Can you work these out from the model? Positions are in its coordinate system, mm. Give positions to 0.01 mm unless a question says otherwise; leave off trailing zeros. Order: outer loops, then holes, each group sorted by start corner. A loop starts at its lowest first (then second) coordinate and runs counter-clockwise, first axis right, second up. Notation, with made-up numbers: (-32, 34.25) -> (-10, 34.25) arc R25 ccw to (-10, 50.25) -> close; hole circle Ø4 at (-40, 33). An arc over 180 degrees is marked (long way). Answer as a JSON object with one key per item and string values.
```python
from build123d import *

# Parameters (mm, degrees)
PLATE_W                                        = 50
PLATE_H                                        = 50
BOSS_EXTRUDE1_DEPTH                            = 3
CSK_FOR_M3_OVAL_HEAD_MACHINE_SCREW1_AT_2_COUNT = 2
CSK_FOR_M3_OVAL_HEAD_MACHINE_SCREW1_AT_2_PITCH = 42
CSK_FOR_M3_OVAL_HEAD_MACHINE_SCREW1_AT_3_COUNT = 2
CSK_FOR_M3_OVAL_HEAD_MACHINE_SCREW1_AT_3_PITCH = 59.39696962
CSK_FOR_M3_OVAL_HEAD_MACHINE_SCREW1_AT_4_COUNT = 2
CSK_FOR_M3_OVAL_HEAD_MACHINE_SCREW1_AT_4_PITCH = 42
F_24_0_24_DIAMETER_HOLE1_D                     = 24
F_24_0_24_DIAMETER_HOLE1_ON_FACE_2_D           = 24
F_24_0_24_DIAMETER_HOLE1_ON_FACE_3_D           = 24
CSK_FOR_M3_OVAL_HEAD_MACHINE_SCREW2_AT_2_COUNT = 2
CSK_FOR_M3_OVAL_HEAD_MACHINE_SCREW2_AT_2_PITCH = 31
CSK_FOR_M3_OVAL_HEAD_MACHINE_SCREW2_AT_3_COUNT = 2
CSK_FOR_M3_OVAL_HEAD_MACHINE_SCREW2_AT_3_PITCH = 43.840620434
CSK_FOR_M3_OVAL_HEAD_MACHINE_SCREW2_AT_4_COUNT = 2
CSK_FOR_M3_OVAL_HEAD_MACHINE_SCREW2_AT_4_PITCH = 31


with BuildPart() as part:
    # Plate → Boss-Extrude1 (new body)
    with BuildSketch(Plane(origin=(0, 0, 0), x_dir=(1, 0, 0), z_dir=(0, 1, 0))):
        Rectangle(PLATE_W, PLATE_H)
    extrude(amount=BOSS_EXTRUDE1_DEPTH)

    # Sketch3 → CSK for M3 Oval Head Machine Screw1 (revolve, cut)
    with BuildSketch(Plane(origin=(-21, 3, 21), x_dir=(0, 0, 1), z_dir=(1, 0, 0))):
        Polygon((0, 0), (0, 3), (1.8, 3), (1.8, 1.35), (3.15, 0), align=None)
    csk_for_m3_oval_head_machine_screw1 = revolve(axis=Axis((-21, 9.35, 21), (0, -1, 0)), mode=Mode.SUBTRACT)

    # CSK for M3 Oval Head Machine Screw1 at 2: CSK for M3 Oval Head Machine Screw1 ×2
    with Locations(*[(0, 0, -i * CSK_FOR_M3_OVAL_HEAD_MACHINE_SCREW1_AT_2_PITCH) for i in range(1, CSK_FOR_M3_OVAL_HEAD_MACHINE_SCREW1_AT_2_COUNT)]):
        add(csk_for_m3_oval_head_machine_screw1, mode=Mode.SUBTRACT)

    # CSK for M3 Oval Head Machine Screw1 at 3: CSK for M3 Oval Head Machine Screw1 ×2
    with Locations(*[Vector(0.707106781, 0, -0.707106781) * (i * CSK_FOR_M3_OVAL_HEAD_MACHINE_SCREW1_AT_3_PITCH) for i in range(1, CSK_FOR_M3_OVAL_HEAD_MACHINE_SCREW1_AT_3_COUNT)]):
        add(csk_for_m3_oval_head_machine_screw1, mode=Mode.SUBTRACT)

    # CSK for M3 Oval Head Machine Screw1 at 4: CSK for M3 Oval Head Machine Screw1 ×2
    with Locations(*[(i * CSK_FOR_M3_OVAL_HEAD_MACHINE_SCREW1_AT_4_PITCH, 0, 0) for i in range(1, CSK_FOR_M3_OVAL_HEAD_MACHINE_SCREW1_AT_4_COUNT)]):
        add(csk_for_m3_oval_head_machine_screw1, mode=Mode.SUBTRACT)

    # Ø24.0 (24) Diameter Hole1 (through all)
    with Locations(Plane.ZX.offset(3)):
        with Locations((0, 0)):
            Hole(F_24_0_24_DIAMETER_HOLE1_D / 2)

    # Ø24.0 (24) Diameter Hole1 on face 2 (through all)
    with Locations(Plane(origin=(0, 0, 0), x_dir=(0, 0, -1), z_dir=(0, -1, 0))):
        with Locations((0, 0)):
            Hole(F_24_0_24_DIAMETER_HOLE1_ON_FACE_2_D / 2)

    # Ø24.0 (24) Diameter Hole1 on face 3 (through all)
    with Locations(Plane(origin=(-62.061079299, -166.048748064, 0), x_dir=(0, 0, 1), z_dir=(0, 1, 0))):
        with Locations((0, 0)):
            Hole(F_24_0_24_DIAMETER_HOLE1_ON_FACE_3_D / 2)

    # Sketch6 → CSK for M3 Oval Head Machine Screw2 (revolve, cut)
    with BuildSketch(Plane(origin=(-15.5, 3, -15.5), x_dir=(0, 0, 1), z_dir=(1, 0, 0))):
        Polygon((0, 0), (0, 3), (1.8, 3), (1.8, 1.35), (3.15, 0), align=None)
    csk_for_m3_oval_head_machine_screw2 = revolve(axis=Axis((-15.5, 9.35, -15.5), (0, -1, 0)), mode=Mode.SUBTRACT)

    # CSK for M3 Oval Head Machine Screw2 at 2: CSK for M3 Oval Head Machine Screw2 ×2
    with Locations(*[(i * CSK_FOR_M3_OVAL_HEAD_MACHINE_SCREW2_AT_2_PITCH, 0, 0) for i in range(1, CSK_FOR_M3_OVAL_HEAD_MACHINE_SCREW2_AT_2_COUNT)]):
        add(csk_for_m3_oval_head_machine_screw2, mode=Mode.SUBTRACT)

    # CSK for M3 Oval Head Machine Screw2 at 3: CSK for M3 Oval Head Machine Screw2 ×2
    with Locations(*[Vector(0.707106781, 0, 0.707106781) * (i * CSK_FOR_M3_OVAL_HEAD_MACHINE_SCREW2_AT_3_PITCH) for i in range(1, CSK_FOR_M3_OVAL_HEAD_MACHINE_SCREW2_AT_3_COUNT)]):
        add(csk_for_m3_oval_head_machine_screw2, mode=Mode.SUBTRACT)

    # CSK for M3 Oval Head Machine Screw2 at 4: CSK for M3 Oval Head Machine Screw2 ×2
    with Locations(*[(0, 0, i * CSK_FOR_M3_OVAL_HEAD_MACHINE_SCREW2_AT_4_PITCH) for i in range(1, CSK_FOR_M3_OVAL_HEAD_MACHINE_SCREW2_AT_4_COUNT)]):
        add(csk_for_m3_oval_head_machine_screw2, mode=Mode.SUBTRACT)


solid = part.part
```
1. If we section it at A-A on z = 21: Please give me the cut outline in (x, y).
Worked answers:
{"outline": "(-25, 0) -> (-22.8, 0) -> (-22.8, 1.65) -> (-24.15, 3) -> (-25, 3) -> close; (-19.2, 0) -> (19.2, 0) -> (19.2, 1.65) -> (17.85, 3) -> (-17.85, 3) -> (-19.2, 1.65) -> close; (22.8, 0) -> (25, 0) -> (25, 3) -> (24.15, 3) -> (22.8, 1.65) -> close"}
2. If we mould it in two halves opening along X, with no side actions, what happens to faces 1 (the face through (-17.285, 0.837, 15.266)), 2 (the face through (-6, 0, -11)), 3 (the face through (-25, 1, 0)), 4 (the face through (19.215, 0.837, 20.766))? For each: +X half, -X half, draft (parallel to the pull), parting line (faces both ways), or undercut.
Worked answers:
{"face 1": "undercut", "face 2": "draft", "face 3": "-X half", "face 4": "undercut"}
3. If we section it at C-C on y = 0.9: Count the separate pieces of the cut face and the enclosed holes in it, then the cut area to 3 significant figures.
Worked answers:
{"separate pieces": "1", "enclosed holes": "9", "area": "1,970 mm²"}
4. If we section it at D-D on z = 0: Please give me the cut outline in (x, y), then the cut area to 3 significant figures.
Worked answers:
{"outline": "(-25, 0) -> (-12, 0) -> (-12, 3) -> (-25, 3) -> close; (12, 0) -> (25, 0) -> (25, 3) -> (12, 3) -> close", "area": "78.0 mm²"}
5. Will these pins go through, and if not, where does the flat tip stop? pin 1 Ø4 at (x, z) = (15.5, -15.5) entering from +Y; pin 2 Ø6 at (x, z) = (21, 21) entering from +Y.
Worked answers:
{"pin 1": "y = 1.85", "pin 2": "y = 2.85"}
6. If we section it at B-B on x = -21: Please give me the cut outline in (y, z), then the cut area to 3 significant figures.
Worked answers:
{"outline": "(0, -25) -> (3, -25) -> (3, -24.15) -> (1.65, -22.8) -> (0, -22.8) -> close; (0, -19.2) -> (1.65, -19.2) -> (3, -17.85) -> (3, 17.85) -> (1.65, 19.2) -> (0, 19.2) -> close; (0, 22.8) -> (1.65, 22.8) -> (3, 24.15) -> (3, 25) -> (0, 25) -> close", "area": "125 mm²"}
7. Please list where these lines run through material, in increasing order: L1, parallel to X at y = 1.1, z = 21; L2, parallel to X at y = 0.55, z = -15.5.
Worked answers:
{"L1": "-25 to -22.8, -19.2 to 19.2, 22.8 to 25", "L2": "-25 to -17.3, -13.7 to 13.7, 17.3 to 25"}
